Work out the finished part from the listing and answer in its coordinate system (mm). Face numbers are marked on the shaded views. A direction names the side the tool comes from. Give positions to 0.01 mm unless a question says otherwise; leave off trailing zeros. Write each loop counter-clockwise with the first axis right and the second up, starting at its lowest first coordinate (ties: lowest second). Pieces come first, ordered by that corner, then holes.
1) Straight lines are drawn through the part: probe 1 along Y at (x, z) = (0, 6); probe 2 along Y at (x, z) = (0.5, 0.75); probe 3 along Z at (x, y) = (3, 1.5). For each, find the intervals that lie inside material, in ascending order.
2) Find section B-B (y = -1.75). Determine the outline of the cut face in (x, z), plus the area to 3 significant figures.
3) Given pin 1 Ø1.5 at (y, z) = (-2.5, 4) entering from +X; pin 2 Ø0.8 at (x, y) = (0.5, 0.5) entering from +Z, each flat-ended and moving along its own axis, determine where each tip first touches the part or whether it passes through.
4) Find section D-D (x = 1.75). Determine the outline of the cut face in (y, z).
5) A tool of negligible diameter and unlimited length cuts with its end or side. For the marked faces 4 and 5, from which of +Z, -Z, +X, -X, +Y, -Y can it reach the whole face along a straight path? Write none if from no direction.
6) Find section C-C (z = 3.25). Determine the outline of the cut face in (x, y), plus the area to 3 significant figures.
7) Find section A-A (x = 0). Determine the outline of the cut face in (y, z).
8) Determine the mould class of the marked faces 1, 2 and 3 for opening direction X: pulls with the +X half, pulls with the -X half, needs draft (parallel to the pull), parting line crosses it, or undercut.
```python
from build123d import *

# Parameters (mm, degrees)
SKETCH_1_R      = 2.5
SKETCH_1_R_2    = 1.25
EXTRUDE_1_DEPTH = 8
EXTRUDE_2_DEPTH = 1


with BuildPart() as part:
    # 草图1 → 凸台-拉伸1 (new body)
    with BuildSketch(Plane.XY):
        Circle(SKETCH_1_R)
        Circle(SKETCH_1_R_2, mode=Mode.SUBTRACT)
    extrude(amount=EXTRUDE_1_DEPTH)

    # 草图2 → 凸台-拉伸2 (add)
    with BuildSketch(Plane(origin=(0, 0, 0), x_dir=(-1, 0, 0), z_dir=(0, 0, -1))):
        Polygon((-2.020725942, -3.5), (2.020725942, -3.5), (4.041451884, 0), (2.020725942, 3.5), (-2.020725942, 3.5), (-4.041451884, 0), align=None)
    extrude(amount=EXTRUDE_2_DEPTH)


solid = part.part
```
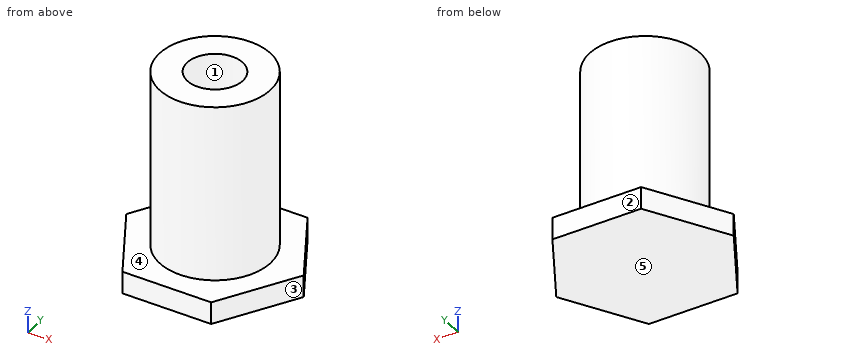
Results:
1. probe 1: y = -2.5 to -1.25, 1.25 to 2.5
1. probe 2: y = -2.45 to -1.15, 1.15 to 2.45
1. probe 3: z = -1 to 0
2. outline: (-3.03, -1) - (3.03, -1) - (3.03, 0) - (1.79, 0) - (1.79, 8) - (-1.79, 8) - (-1.79, 0) - (-3.03, 0) - close
2. area: 34.6 mm2
3. pin 1: stops at x = 1.79
3. pin 2: stops at z = 0
4. outline: (-3.5, -1) - (3.5, -1) - (3.5, 0) - (1.79, 0) - (1.79, 8) - (-1.79, 8) - (-1.79, 0) - (-3.5, 0) - close
5. face 4: +Z
5. face 5: -Z, +X, -X, +Y, -Y
6. outline: circle Ø5 at (0, 0); hole circle Ø2.5 at (0, 0)
6. area: 14.7 mm2
7. outline: (-3.5, -1) - (3.5, -1) - (3.5, 0) - (2.5, 0) - (2.5, 8) - (1.25, 8) - (1.25, 0) - (-1.25, 0) - (-1.25, 8) - (-2.5, 8) - (-2.5, 0) - (-3.5, 0) - close
8. face 1: undercut
8. face 2: needs draft
8. face 3: pulls with the +X half
